Read the model definition and answer for the solid it produces. Units are mm, in the model's axes. A direction names the side the tool comes from. Coordinates: 2 decimals unless noted, no trailing zeros. Loops run counter-clockwise (first coordinate to the right, second up) from the corner with the lowest first, then second, coordinate; pieces in that order, holes last.
from build123d import *

# Parameters (mm, degrees)
SKETCH1_W           = 44.45
SKETCH1_H           = 44.45
SKETCH1_W_2         = 38.1
SKETCH1_H_2         = 38.1
BOSS_EXTRUDE1_DEPTH = 1981.2
SKETCH2_R           = 18.25625
CUT_EXTRUDE1_DEPTH  = 45.45
SKETCH3_R           = 4.7625
CUT_EXTRUDE2_DEPTH  = 45.45


with BuildPart() as part:
    # Sketch1 → Boss-Extrude1 (new body)
    with BuildSketch(Plane(origin=(0, 0, 0), x_dir=(1, 0, 0), z_dir=(0, 1, 0))):
        with Locations((22.225, 22.225)):
            Rectangle(SKETCH1_W, SKETCH1_H)
        with Locations((22.225, 22.225)):
            Rectangle(SKETCH1_W_2, SKETCH1_H_2, mode=Mode.SUBTRACT)
    extrude(amount=BOSS_EXTRUDE1_DEPTH)

    # Sketch2 → Cut-Extrude1 (cut, through all)
    with BuildSketch(Plane.XY):
        with Locations((22.225, 22.225)):
            Circle(SKETCH2_R)
        with Locations((22.225, 911.225)):
            Circle(SKETCH2_R)
    extrude(amount=-CUT_EXTRUDE1_DEPTH, mode=Mode.SUBTRACT)

    # Sketch3 → Cut-Extrude2 (cut, through all)
    with BuildSketch(Plane(origin=(44.45, 0, 0), x_dir=(0, 0, -1), z_dir=(1, 0, 0))):
        with Locations((22.225, 22.225)):
            Circle(SKETCH3_R)
        with Locations((22.225, 911.225)):
            Circle(SKETCH3_R)
    extrude(amount=-CUT_EXTRUDE2_DEPTH, mode=Mode.SUBTRACT)


solid = part.part
Item 1: A cutting plane is placed at A-A on z = -10. Determine the outline of the cut face in (x, y) (3 decimals).
Numbers:
outline: (0, 0) - (3.175, 0) - (3.175, 1981.2) - (0, 1981.2) - close; (41.275, 0) - (44.45, 0) - (44.45, 1981.2) - (41.275, 1981.2) - close
Item 2: A cutting plane is placed at B-B on y = 1340. Determine the outline of the cut face in (x, z) (3 decimals).
Numbers:
outline: (0, -44.45) - (44.45, -44.45) - (44.45, 0) - (0, 0) - close; hole (3.175, -41.275) - (41.275, -41.275) - (41.275, -3.175) - (3.175, -3.175) - close
Item 3: Find the intervals of material crossed by line 1 along Z through (x, y) = (23.5, 1688) (3 decimals); line 2 along X through (y, z) = (140, -9) (3 decimals), in increasing order.
Numbers:
line 1: z = -44.45 to -41.275, -3.175 to 0
line 2: x = 0 to 3.175, 41.275 to 44.45
Item 4: Determine the mould class of faces 1 (the face through (30.65, 6.03, -42.84)), 2 (the face through (42, 1981.2, -23)), 3 (the face through (42, 0, -23)), 4 (the face through (3.175, 977, -22)) for opening direction Y: released by +Y, released by -Y, zero draft, split by the parting line, or undercut.
Numbers:
face 1: undercut
face 2: released by +Y
face 3: released by -Y
face 4: zero draft
Item 5: Given pin 1 (5 mm diameter, centred on x = 33.5, y = 297.5, fed in from +Z); pin 2 (8.5 mm diameter, centred on y = 22.225, z = -22.225, fed in from +X), each flat-ended and moving along its own axis, determine where each tip first touches the part or whether it passes through.
Numbers:
pin 1: stops at z = 0
pin 2: passes through
Item 6: Which of the six approach directions +Z, -Z, +X, -X, +Y, -Y give full straight-line access (tool end or side, diameter ignored) to faces 5 (the face through (0, 977, -22)), 6 (the face through (22, 977, -3.175))?
Numbers:
face 5: +Z, -Z, -X, +Y, -Y
face 6: +Y, -Y
Item 7: A cutting plane is placed at C-C on x = 31.5. Determine the outline of the cut face in (y, z) (3 decimals), then the cut area to 3 significant figures.
Numbers:
outline: (0, -44.45) - (6.5, -44.45) - (6.5, -41.275) - (0, -41.275) - close; (0, -3.175) - (6.5, -3.175) - (6.5, 0) - (0, 0) - close; (37.95, -44.45) - (895.5, -44.45) - (895.5, -41.275) - (37.95, -41.275) - close; (37.95, -3.175) - (895.5, -3.175) - (895.5, 0) - (37.95, 0) - close; (926.95, -44.45) - (1981.2, -44.45) - (1981.2, -41.275) - (926.95, -41.275) - close; (926.95, -3.175) - (1981.2, -3.175) - (1981.2, 0) - (926.95, 0) - close
area: 12,200 mm2
